Verification items for the finished model (mm, model axes). Face numbers are marked on the shaded views. A direction names the side the tool comes from. Give positions to 0.01 mm unless a question says otherwise; leave off trailing zeros. Loops run counter-clockwise (first coordinate to the right, second up) from the corner with the lowest first, then second, coordinate; pieces in that order, holes last. Notation, with made-up numbers: M -32,-14 L 12,-14 A20 cw 12,6 Z; hole C 75,69 d7. An arc over 180 degrees is marked long. Put each result on its own line as item: value. Start each with the question number.
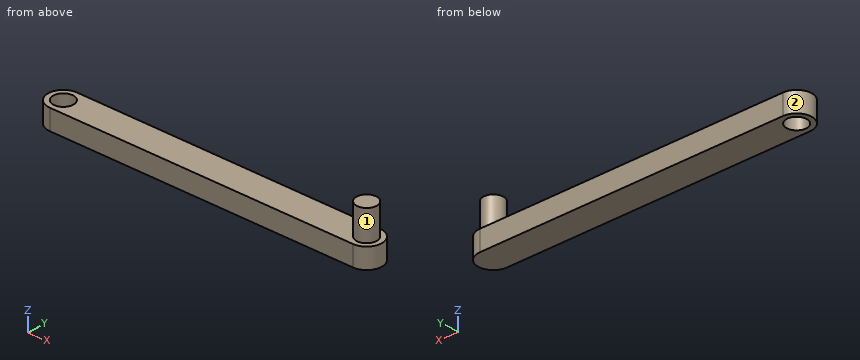
Autodesk Inventor part; units mm, degrees
ref_plane "YZ Plane" through (0, 0, 0) normal (1, 0, 0) x (0, 1, 0)
ref_plane "XZ Plane" through (0, 0, 0) normal (0, 1, 0) x (-1, 0, 0)
ref_plane "XY Plane" through (0, 0, 0) normal (0, 0, 1) x (1, 0, 0)
sketch "Sketch1" plane through (0, 0, 0) normal (0, 0, 1) x (1, 0, 0)
  line L0 (-110.5069, 7.5) -> (39.4931, 7.5)
  line L1 (39.4931, 7.5) -> (39.4931, -7.5)
  line L2 (39.4931, -7.5) -> (-110.5069, -7.5)
  line L3 (-110.5069, -7.5) -> (-110.5069, 7.5)
  arc A0 (-110.5069, 7.5) -> (-110.5069, -7.5) centre (-110.5069, 0) ccw
  arc A1 (39.4931, -7.5) -> (39.4931, 7.5) centre (39.4931, 0) ccw
  circle A2 centre (-110.5069, 0) radius 5
  point P0 (0, 0)
  dimension "d0" = 150
  dimension "d1" = 15
  dimension "d2" = 7.5
  dimension "d3" = 10
extrude "Extrusion1" add sketch "Sketch1" along normal blind 10 contours L0 L1 L2 L3 A2 | L3 A2 A0 | A1 L1
sketch "Sketch2" plane through (0, 0, 10) normal (0, 0, 1) x (1, 0, 0)
  arc A0 (39.4931, -7.5) -> (39.4931, 7.5) centre (39.4931, 0) ccw
  circle A1 centre (39.4931, 0) radius 5
  point P0 (0, 0)
  dimension "d6" = 10
extrude "Extrusion2" add sketch "Sketch2" along normal blind 15
properties part number "innerLink" material "Stainless Steel"
Q1. Cross-section at A-A, the plane y = 0. Record the boundary of the cut face in (x, z), then the cut area to 3 significant figures.
Q2. Cross-section at C-C, the plane x = 2.5. Record the boundary of the cut face in (y, z), then the cut area to 3 significant figures.
Q3. Go/stop test with flat-tipped pins: pin 1 (4 mm diameter, centred on y = -4.5, z = 8, fed in from -X); pin 2 (4 mm diameter, centred on y = -4, z = 7.5, fed in from +X); pin 3 (4.5 mm diameter, centred on x = -76.5, y = 1.5, fed in from +Z). Record where each tip stops, or that it passes through.
Q4. Cross-section at B-B, the plane z = 12.25. Record the boundary of the cut face in (x, y), then the cut area to 3 significant figures.
Q5. Scan lines: L1, parallel to X at y = 0, z = 6.5; L2, parallel to Z at x = 17, y = 4.75; L3, parallel to X at y = -1, z = 6.5. Record each from-to range of solid material in increasing order.
Q6. Set-up check for the marked faces 1 and 2: record each of +Z, -Z, +X, -X, +Y, -Y from which the full face is reachable in a straight line by a thin tool's end or side.
Ans:
1. outline: M -118.01,0 L -115.51,0 L -115.51,10 L -118.01,10 Z; M -105.51,0 L 46.99,0 L 46.99,10 L 44.49,10 L 44.49,25 L 34.49,25 L 34.49,10 L -105.51,10 Z
1. area: 1,700 mm^2
2. outline: M -7.5,0 L 7.5,0 L 7.5,10 L -7.5,10 Z
2. area: 150 mm^2
3. pin 1: stops at x = -117.58
3. pin 2: stops at x = 46.72
3. pin 3: stops at z = 10
4. outline: C 39.49,0 d10
4. area: 78.5 mm^2
5. L1: x = -118.01 to -115.51, -105.51 to 46.99
5. L2: z = 0 to 10
5. L3: x = -117.94 to -115.41, -105.61 to 46.93
6. face 1: +Z
6. face 2: +Z, -Z, -X
